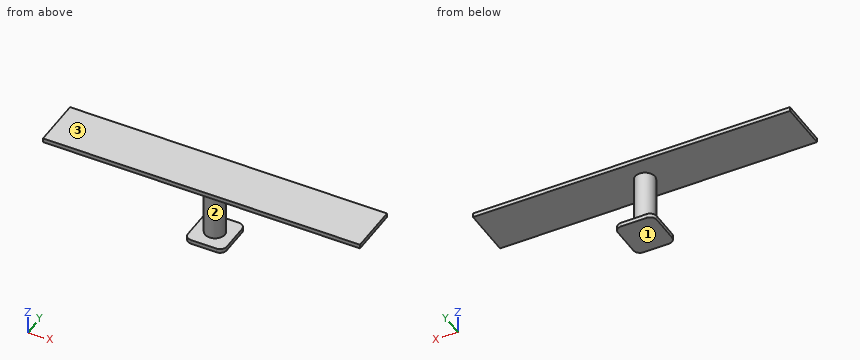
Autodesk Inventor part; units mm, degrees
ref_plane "YZ Plane" through (0, 0, 0) normal (1, 0, 0) x (0, 1, 0)
ref_plane "XZ Plane" through (0, 0, 0) normal (0, 1, 0) x (-1, 0, 0)
ref_plane "XY Plane" through (0, 0, 0) normal (0, 0, 1) x (1, 0, 0)
sketch "Sketch1" plane through (0, 0, 0) normal (0, 0, 1) x (1, 0, 0)
  line L0 (-2.2587, 5.9544) -> (9.9913, 5.9544)
  line L1 (13.1663, 2.7794) -> (13.1663, -10.8706)
  line L2 (9.9913, -14.0456) -> (-2.2587, -14.0456)
  line L3 (-5.4337, -10.8706) -> (-5.4337, 2.7794)
  arc A0 (13.1663, 2.7794) -> (9.9913, 5.9544) centre (9.9913, 2.7794) ccw
  arc A1 (9.9913, -14.0456) -> (13.1663, -10.8706) centre (9.9913, -10.8706) ccw
  arc A2 (-5.4337, -10.8706) -> (-2.2587, -14.0456) centre (-2.2587, -10.8706) ccw
  arc A3 (-2.2587, 5.9544) -> (-5.4337, 2.7794) centre (-2.2587, 2.7794) ccw
  point P0 (0, 0)
  point P1 (13.1663, -14.0456)
  point P2 (13.1663, 5.9544)
  point P3 (-5.4337, -14.0456)
  dimension "d0" = 18.6
  dimension "d1" = 20
  dimension "d2" = 3.175
extrude "Extrusion1" add sketch "Sketch1" along normal blind 2
sketch "Sketch2" plane through (0, 0, 2) normal (0, 0, 1) x (1, 0, 0)
  arc A0 (-2.2587, 5.9544) -> (-5.4337, 2.7794) centre (-2.2587, 2.7794) ccw
  arc A1 (9.9913, -14.0456) -> (13.1663, -10.8706) centre (9.9913, -10.8706) ccw
  line L0 (-2.2587, 2.7794) -> (9.9913, -10.8706) construction
  arc A2 (13.1663, 2.7794) -> (9.9913, 5.9544) centre (9.9913, 2.7794) ccw
  arc A3 (-5.4337, -10.8706) -> (-2.2587, -14.0456) centre (-2.2587, -10.8706) ccw
  line L1 (9.9913, 2.7794) -> (-2.2587, -10.8706) construction
  circle A4 centre (3.8663, -4.0456) radius 4.7625
  point P0 (0, 0)
  dimension "d5" = 9.525
extrude "Extrusion2" add sketch "Sketch2" along normal blind 28
sketch "Sketch3" plane through (3.8663, -4.0456, 30) normal (0, 0, 1) x (1, 0, 0)
  line L0 (-76.2, -12.065) -> (76.2, -12.065)
  line L1 (76.2, -12.065) -> (76.2, 12.065)
  line L2 (76.2, 12.065) -> (-76.2, 12.065)
  line L3 (-76.2, 12.065) -> (-76.2, -12.065)
  line L4 (-76.2, -12.065) -> (76.2, 12.065) construction
  line L5 (76.2, -12.065) -> (-76.2, 12.065) construction
  point P0 (-3.8663, 4.0456)
  point P1 (0, 0)
  point P2 (0, 0)
  dimension "d8" = 24.13
  dimension "d9" = 152.4
extrude "Extrusion3" add sketch "Sketch3" along normal blind 2
properties part number "Hot Shoe Mount"
Geometry: final body of the model. Coordinates: model frame, mm. Face numbers are marked on the shaded views. Coordinates: 2 decimals unless noted, no trailing zeros. Loops run counter-clockwise (first coordinate to the right, second up) from the corner with the lowest first, then second, coordinate; pieces in that order, holes last. Notation, with made-up numbers: M 62,-5.75 L 76,-5.75 A26 cw 76,17.25 Z; hole C 76.25,15 d6. An arc over 180 degrees is marked long. Put each result on its own line as item: value.
(1) Draft query along Z for the marked faces 1, 2 and 3. Return one class per face: pulls with the +Z half, pulls with the -Z half, needs draft (parallel to the pull), parting line crosses it, or undercut.
Answer sheet:
face 1: pulls with the -Z half
face 2: undercut
face 3: pulls with the +Z half
(2) Cut plane C-C on z = 18. Return the cut outline in (x, y) (1 decimal).
Answer sheet:
outline: C 3.9,-4 d9.5
(3) First-contact query: pin 1 (4 mm diameter, centred on x = -41, y = -5.5, fed in from -Z); pin 2 (2 mm diameter, centred on y = -2.5, z = 1, fed in from -X); pin 3 (1.6 mm diameter, centred on x = 2, z = 1, fed in from +Y). Flat tips, straight axial feed; report the tip coordinate or a pass-through.
Answer sheet:
pin 1: stops at z = 30
pin 2: stops at x = -5.43
pin 3: stops at y = 5.95
(4) Material intervals for probe 1 along Z at (x, y) = (11.5, -8.5); probe 2 along Z at (x, y) = (39.5, 0); probe 3 along X at (y, z) = (-0.5, 19), sorted ascending.
Answer sheet:
probe 1: z = 0 to 2, 30 to 32
probe 2: z = 30 to 32
probe 3: x = 0.69 to 7.05
(5) Cut plane A-A on y = -7. Return the cut outline in (x, z).
Answer sheet:
outline: M -72.33,30 L 0.13,30 L 0.13,2 L -5.43,2 L -5.43,0 L 13.17,0 L 13.17,2 L 7.6,2 L 7.6,30 L 80.07,30 L 80.07,32 L -72.33,32 Z
(6) Cut plane B-B on x = 3. Return the cut outline in (y, z).
Answer sheet:
outline: M -16.11,30 L -8.73,30 L -8.73,2 L -14.05,2 L -14.05,0 L 5.95,0 L 5.95,2 L 0.64,2 L 0.64,30 L 8.02,30 L 8.02,32 L -16.11,32 Z
